```python
from build123d import *

# Parameters (mm, degrees)
F0_W     = 23.6982
F0_H     = 15.7734
F1_DEPTH = 9.5377
F2_R     = 2.44475
F3_DEPTH = 1.778
F4_W     = 21.4122
F4_H     = 13.4874
F4_R     = 3.2385
F5_DEPTH = 8.382
F4_R_2   = 2.33045
F6_DEPTH = 8.382


with BuildPart() as f1:
    # F0 (on Top) → F1 (new body)
    with BuildSketch(Plane.XY):
        Rectangle(F0_W, F0_H)
    extrude(amount=F1_DEPTH)

    # F2 (on face) → F3 (join)
    with BuildSketch(Plane.XY.offset(9.5377)):
        with Locations((-8.04545, -4.08305)):
            Circle(F2_R)
        with Locations((0, -4.08305)):
            Circle(F2_R)
        with Locations((8.04545, -4.08305)):
            Circle(F2_R)
        with Locations((8.04545, 4.08305)):
            Circle(F2_R)
        with Locations((0, 4.08305)):
            Circle(F2_R)
        with Locations((-8.04545, 4.08305)):
            Circle(F2_R)
    extrude(amount=F3_DEPTH)

    # F4 (on face) → F5 (cut)
    with BuildSketch(Plane(origin=(0, 0, 0), x_dir=(1, 0, 0), z_dir=(0, 0, -1))):
        Rectangle(F4_W, F4_H)
        with Locations((-6.298674, 0)):
            Circle(F4_R, mode=Mode.SUBTRACT)
        with Locations((5.322928, 0)):
            Circle(F4_R, mode=Mode.SUBTRACT)
    extrude(amount=-F5_DEPTH, mode=Mode.SUBTRACT)

    # F4 (on face) → F6 (cut)
    with BuildSketch(Plane(origin=(0, 0, 0), x_dir=(1, 0, 0), z_dir=(0, 0, -1))):
        with Locations((-6.298674, 0)):
            Circle(F4_R_2)
        with Locations((5.322928, 0)):
            Circle(F4_R_2)
    extrude(amount=-F6_DEPTH, mode=Mode.SUBTRACT)


solid = f1.part
```
CAD build for the part. Positions are in the model's coordinates, mm. A direction names the side the tool comes from. Coordinates: 2 decimals unless noted, no trailing zeros. Write each loop counter-clockwise with the first axis right and the second up, starting at its lowest first coordinate (ties: lowest second). Pieces come first, ordered by that corner, then holes. Notation, with made-up numbers: (58, 54) -> (113, 54) arc R18 ccw to (113, 72) -> close; hole circle Ø11 at (62, 24.25). An arc over 180 degrees is marked (long way). Return JSON: item names as keys, results as strings. Group by question number.
Q1. Flat gauge pins, fed straight in: pin 1 (7.5 mm diameter, centred on x = 5.32, y = 0, fed in from -Z); pin 2 (2.5 mm diameter, centred on x = -6, y = 0, fed in from -Z). Where does each tip first touch, or does it go through?
Q2. Cut at A-A, the plane z = 6. Give the cut face in (x, y).
Q3. Drill centre lines: line 1 (X direction, y = 0, z = 2.5); line 2 (Y direction, x = -2.25, z = 3.5); line 3 (X direction, y = 6, z = 7). Where is each one in solid material? Low to high.
Q4. Cut at D-D, the plane z = 10. Give the cut face in (x, y), then the cut area to 3 significant figures.
Q5. Cut at B-B, the plane y = 0. Give the cut face in (x, z).
Q6. Pull direction X, two halves, no side cores. Call faces 1 (the face through (-11.849, 0, 5)), 2 (the face through (-6, 0, 8.382)), 3 (the face through (-1, -7, 0)): released by +X, released by -X, zero draft, split by the parting line, or undercut.
Q7. Cut at C-C, the plane x = -2.75. Give the cut face in (y, z), then the cut area to 3 significant figures.
Q8. Which spindle directions (+Z, -Z, +X, -X, +Y, -Y) get a long thin tool onto all of the face, cutting with end or side? Do faces 4 (the face through (8.314, 1.24, 4.132)), 5 (the face through (-8, 4, 11.316)), 6 (the face through (6.105, -5.571, 10.414)). Say none if no direction does.
Returned:
{
 "1": {"pin 1": "stops at z = 0", "pin 2": "stops at z = 8.38"},
 "2": {"outline": "(-11.85, -7.89) -> (11.85, -7.89) -> (11.85, 7.89) -> (-11.85, 7.89) -> close; circle Ø6.48 at (-6.3, 0); circle Ø6.48 at (5.32, 0); hole (-10.71, -6.74) -> (10.71, -6.74) -> (10.71, 6.74) -> (-10.71, 6.74) -> close; hole circle Ø4.66 at (-6.3, 0); hole circle Ø4.66 at (5.32, 0)"},
 "3": {"line 1": "x = -11.85 to -10.71, -9.54 to -8.63, -3.97 to -3.06, 2.08 to 2.99, 7.65 to 8.56, 10.71 to 11.85", "line 2": "y = -7.89 to -6.74, 6.74 to 7.89", "line 3": "x = -11.85 to -10.71, 10.71 to 11.85"},
 "4": {"outline": "circle Ø4.89 at (-8.05, -4.08); circle Ø4.89 at (-8.05, 4.08); circle Ø4.89 at (0, -4.08); circle Ø4.89 at (0, 4.08); circle Ø4.89 at (8.05, -4.08); circle Ø4.89 at (8.05, 4.08)", "area": "113 mm2"},
 "5": {"outline": "(-11.85, 0) -> (-10.71, 0) -> (-10.71, 8.38) -> (-9.54, 8.38) -> (-9.54, 0) -> (-8.63, 0) -> (-8.63, 8.38) -> (-3.97, 8.38) -> (-3.97, 0) -> (-3.06, 0) -> (-3.06, 8.38) -> (2.08, 8.38) -> (2.08, 0) -> (2.99, 0) -> (2.99, 8.38) -> (7.65, 8.38) -> (7.65, 0) -> (8.56, 0) -> (8.56, 8.38) -> (10.71, 8.38) -> (10.71, 0) -> (11.85, 0) -> (11.85, 9.54) -> (-11.85, 9.54) -> close"},
 "6": {"face 1": "released by -X", "face 2": "undercut", "face 3": "zero draft"},
 "7": {"outline": "(-7.89, 0) -> (-6.74, 0) -> (-6.74, 8.38) -> (6.74, 8.38) -> (6.74, 0) -> (7.89, 0) -> (7.89, 9.54) -> (-7.89, 9.54) -> close", "area": "37.4 mm2"},
 "8": {"face 4": "-Z", "face 5": "+Z, +X, -X, +Y, -Y", "face 6": "+Z"}
}
